from build123d import *

# Parameters (mm, degrees)
F0_R          = 14
F1_DEPTH      = 30
F2_T          = -5
F3_R          = 3.5
F4_DEPTH      = 14.001
F4_DEPTH_BACK = 14.001


# Not quite as in the source:
# - a fillet or chamfer that OpenCascade refuses, or shapes differently, is made with other operations: its cross-section is extruded or revolved along the edge and cut away or added


with BuildPart() as f1:
    # F0 (on Top) → F1 (new body)
    with BuildSketch(Plane.XY):
        Circle(F0_R)
    extrude(amount=F1_DEPTH)

    # F2
    f2_openings = [f1.faces().sort_by_distance(p)[0] for p in [
        (0, 0, 0),
    ]]
    offset(amount=F2_T, openings=f2_openings)

    # F3 (on Right) → F4 (cut, two sides)
    with BuildSketch(Plane.YZ) as f4_sk:
        with Locations((0, 10)):
            Circle(F3_R)
    extrude(amount=-F4_DEPTH, mode=Mode.SUBTRACT)
    extrude(f4_sk.sketch, amount=F4_DEPTH_BACK, mode=Mode.SUBTRACT)

    # F5: chamfer of 5.08 on 1 edges, made by hand

    # F5_s1 → F5_t2 (revolve, cut)
    with BuildSketch(Plane.XZ):
        Polygon((14.08, 0), (9, 5.08), (9, 0), align=None)
    revolve(axis=Axis((0, 0, 0), (0, 0, 1)), mode=Mode.SUBTRACT)


solid = f1.part
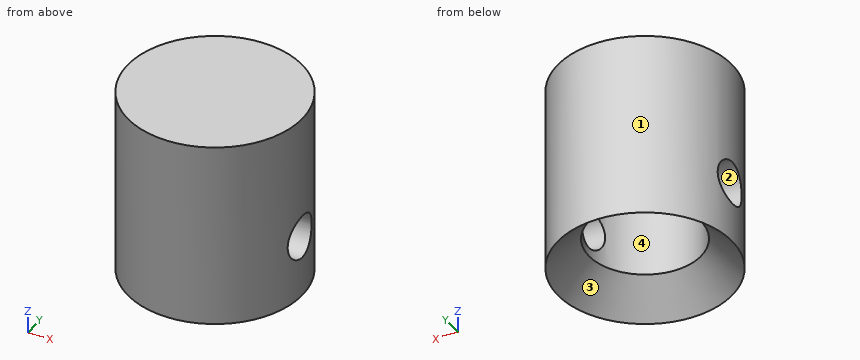
The model under review builds one solid part; all positions refer to its coordinate system, in mm. Face numbers are marked on the shaded views. Round coordinates to 2 decimals unless told otherwise and drop trailing zeros. Loops run counter-clockwise (first coordinate to the right, second up) from the corner with the lowest first, then second, coordinate; pieces in that order, holes last. Notation, with made-up numbers: (63, 40) -> (76, 40) arc R32 cw to (76, 70) -> close; hole circle Ø2 at (-7, -39.75). An arc over 180 degrees is marked (long way). Return JSON: item names as keys, results as strings.
(1) For line 1 (X direction, y = 0, z = 19); line 2 (Z direction, x = 11.3, y = 0); line 3 (Y direction, x = -1.5, z = 17), list the stretches that pass through material, from the lowest coordinate up.
Solved:
{"line 1": "-14 to -9, 9 to 14", "line 2": "2.78 to 6.5, 13.5 to 30", "line 3": "-13.92 to -8.87, 8.87 to 13.92"}
(2) For pin 1 (8 mm diameter, centred on y = 7.5, z = 24.5, fed in from +X); pin 2 (4 mm diameter, centred on x = 2.5, z = 18, fed in from -Y); pin 3 (1 mm diameter, centred on x = 6.5, y = -6.5, fed in from -Z); pin 4 (12 mm diameter, centred on y = -3.5, z = 23, fed in from +X), all flat-tipped, find the tip position at first contact; note any pin that passes through.
Solved:
{"pin 1": "x = 13.56", "pin 2": "y = -13.99", "pin 3": "z = 4.39", "pin 4": "x = 14"}
(3) The part is to be moulded in two halves that separate along X. For the marked faces 1, 2, 3 and 4, say which applies: released by +X, released by -X, zero draft, split by the parting line, or undercut.
Solved:
{"face 1": "split by the parting line", "face 2": "zero draft", "face 3": "undercut", "face 4": "undercut"}
(4) Add section A-A on y = 0. Write out the cut boundary in (x, z).
Solved:
{"outline": "(-14, 0.08) -> (-9, 5.08) -> (-9, 6.5) -> (-14, 6.5) -> close; (-14, 13.5) -> (-9, 13.5) -> (-9, 25) -> (9, 25) -> (9, 13.5) -> (14, 13.5) -> (14, 30) -> (-14, 30) -> close; (9, 5.08) -> (14, 0.08) -> (14, 6.5) -> (9, 6.5) -> close"}
(5) Add section D-D on z = 27.25. Write out the cut boundary in (x, y).
Solved:
{"outline": "circle Ø28 at (0, 0)"}
(6) Add section B-B on z = 7. Write out the cut boundary in (x, y), plus the area to 3 significant figures.
Solved:
{"outline": "(-13.88, -1.8) arc R14 ccw to (13.88, -1.8) -> (8.82, -1.8) arc R9 cw to (-8.82, -1.8) -> close; (-13.88, 1.8) -> (-8.82, 1.8) arc R9 cw to (8.82, 1.8) -> (13.88, 1.8) arc R14 ccw to start", "area": "325 mm2"}
(7) Add section C-C on x = 0. Write out the cut boundary in (y, z).
Solved:
{"outline": "(-14, 0.08) -> (-9, 5.08) -> (-9, 25) -> (9, 25) -> (9, 5.08) -> (14, 0.08) -> (14, 30) -> (-14, 30) -> close"}
